Read the model definition and answer for the solid it produces. Units are mm, in the model's axes. Round coordinates to 2 decimals unless told otherwise and drop trailing zeros. Order: outer loops, then holes, each group sorted by start corner. A loop starts at its lowest first (then second) coordinate and runs counter-clockwise, first axis right, second up.
Autodesk Inventor part; units mm, degrees
ref_plane "YZ Plane" through (0, 0, 0) normal (1, 0, 0) x (0, 1, 0)
ref_plane "XZ Plane" through (0, 0, 0) normal (0, 1, 0) x (-1, 0, 0)
ref_plane "XY Plane" through (0, 0, 0) normal (0, 0, 1) x (1, 0, 0)
sketch "Szkic1" plane through (0, 0, 0) normal (0, 0, 1) x (1, 0, 0)
  line L0 (-236, 32.5) -> (236, 32.5)
  line L1 (236, 32.5) -> (236, -32.5)
  line L2 (236, -32.5) -> (-236, -32.5)
  line L3 (-236, -32.5) -> (-236, 32.5)
  line L4 (-236, 32.5) -> (236, -32.5) construction
  line L5 (236, 32.5) -> (-236, -32.5) construction
  line L6 (-225, -12.5) -> (225, -12.5)
  line L7 (225, -12.5) -> (225, 32.5)
  line L8 (225, 32.5) -> (-225, 32.5)
  line L9 (-225, 32.5) -> (-225, -12.5)
  line L10 (-225, -12.5) -> (225, 32.5) construction
  line L11 (225, -12.5) -> (-225, 32.5) construction
  line L12 (-236, 22.5) -> (-225, 22.5)
  line L13 (-225, 22.5) -> (-225, 2.5)
  line L14 (-225, 2.5) -> (-236, 2.5)
  line L15 (-236, 2.5) -> (-236, 22.5)
  line L16 (225, 22.5) -> (236, 22.5)
  line L17 (236, 22.5) -> (236, 2.5)
  line L18 (236, 2.5) -> (225, 2.5)
  line L19 (225, 2.5) -> (225, 22.5)
  line L20 (-85.5, -12.5) -> (-55.5, -12.5)
  line L21 (-55.5, -12.5) -> (-55.5, -32.5)
  line L22 (-55.5, -32.5) -> (-85.5, -32.5)
  line L23 (-85.5, -32.5) -> (-85.5, -12.5)
  line L24 (-85.5, -12.5) -> (-55.5, -32.5) construction
  line L25 (-55.5, -12.5) -> (-85.5, -32.5) construction
  line L26 (55.5, -12.5) -> (85.5, -12.5)
  line L27 (85.5, -12.5) -> (85.5, -32.5)
  line L28 (85.5, -32.5) -> (55.5, -32.5)
  line L29 (55.5, -32.5) -> (55.5, -12.5)
  line L30 (55.5, -12.5) -> (85.5, -32.5) construction
  line L31 (85.5, -12.5) -> (55.5, -32.5) construction
  line L32 (-76, -23) -> (-65, -23)
  line L33 (-63, -21) -> (-63, -19)
  line L34 (-65, -17) -> (-76, -17)
  line L35 (-78, -19) -> (-78, -21)
  line L36 (-78, -23) -> (-63, -17) construction
  line L37 (-63, -23) -> (-78, -17) construction
  line L38 (65, -17) -> (76, -17)
  line L39 (78, -19) -> (78, -21)
  line L40 (76, -23) -> (65, -23)
  line L41 (63, -21) -> (63, -19)
  line L42 (63, -17) -> (78, -23) construction
  line L43 (78, -17) -> (63, -23) construction
  arc A0 (-65, -23) -> (-63, -21) centre (-65, -21) ccw
  arc A1 (-63, -19) -> (-65, -17) centre (-65, -19) ccw
  arc A2 (-76, -17) -> (-78, -19) centre (-76, -19) ccw
  arc A3 (-78, -21) -> (-76, -23) centre (-76, -21) ccw
  arc A4 (63, -21) -> (65, -23) centre (65, -21) ccw
  arc A5 (65, -17) -> (63, -19) centre (65, -19) ccw
  arc A6 (78, -19) -> (76, -17) centre (76, -19) ccw
  arc A7 (76, -23) -> (78, -21) centre (76, -21) ccw
  line L44 (225, -12.5) -> (195, -12.5)
  line L45 (195, -12.5) -> (195, -6.5)
  line L46 (195, -6.5) -> (225, -6.5)
  line L47 (225, -6.5) -> (225, -12.5)
  line L48 (-225, -12.5) -> (-195, -12.5)
  line L49 (-195, -12.5) -> (-195, -6.5)
  line L50 (-195, -6.5) -> (-225, -6.5)
  line L51 (-225, -6.5) -> (-225, -12.5)
  point P0 (0, 0)
  point P1 (0, 0)
  point P2 (-70.5, -22.5)
  point P3 (70.5, -22.5)
  point P4 (-70.5, -20)
  point P5 (70.5, -20)
  dimension "d0" = 472
  dimension "d1" = 65
  dimension "d2" = 450
  dimension "d3" = 45
  dimension "d4" = 10
  dimension "d5" = 11
  dimension "d6" = 20
  dimension "d7" = 10
  dimension "d8" = 20
  dimension "d9" = 141
  dimension "d10" = 20
  dimension "d11" = 20
  dimension "d12" = 30
  dimension "d13" = 30
  dimension "d15" = 70.5
  dimension "d16" = 15
  dimension "d17" = 6
  dimension "d18" = 4.5
  dimension "d19" = 15
  dimension "d20" = 6
  dimension "d21" = 4.5
  dimension "d22" = 2
  dimension "d25" = 30
  dimension "d26" = 6
  dimension "d27" = 30
  dimension "d28" = 6
extrude "Wyciągnięcie proste1" add sketch "Szkic1" along normal blind 5 contours L0 L7 L46 L45 L6 L49 L50 L9 | L12 L9 L14 L3 | L16 L1 L18 L7 | L23 L6 L21 L2 | L29 L6 L27 L2
equation "\"d21\" = d18"
properties part number "poprz_690"
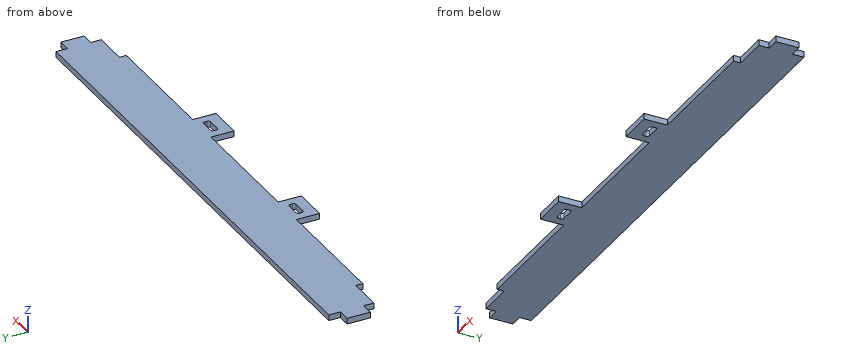
Q1. A cutting plane is placed at A-A, the plane x = 201. Give the vertices of the cut face in (y, z), plus the area to 3 significant figures.
Outcome:
outline: (-6.5, 0) - (32.5, 0) - (32.5, 5) - (-6.5, 5) - close
area: 195 mm2
Q2. Flat-ended cylindrical pins translate along their axes: pin 1 (1.5 mm diameter, centred on y = -24.5, z = 2.5, fed in from +X); pin 2 (1.5 mm diameter, centred on y = -9, z = 3.5, fed in from -X); pin 3 (1.6 mm diameter, centred on y = -20, z = 1.5, fed in from -X). Find the tip coordinate at first contact, or state that the pin passes through.
Outcome:
pin 1: stops at x = 85.5
pin 2: stops at x = -195
pin 3: stops at x = -85.5
Q3. Straight lines are drawn through the part: probe 1 along Y at (x, z) = (-66.5, 2.35); probe 2 along X at (y, z) = (-17.5, 0.3); probe 3 along Y at (x, z) = (-5, 1). For each, find the intervals that lie inside material, in ascending order.
Outcome:
probe 1: y = -32.5 to -23, -17 to 32.5
probe 2: x = -85.5 to -77.32, -63.68 to -55.5, 55.5 to 63.68, 77.32 to 85.5
probe 3: y = -12.5 to 32.5
Q4. A cutting plane is placed at B-B, the plane z = 2.45. Give the number of separate pieces and of enclosed holes in the cut face, plus the area to 3 significant figures.
Outcome:
separate pieces: 1
enclosed holes: 2
area: 21,400 mm2
Q5. A cutting plane is placed at C-C, the plane x = -42. Give the vertices of the cut face in (y, z).
Outcome:
outline: (-12.5, 0) - (32.5, 0) - (32.5, 5) - (-12.5, 5) - close
